from build123d import *

# Parameters (mm, degrees)
BOSS_EXTRUDE1_DEPTH = 40
SKETCH2_W           = 104
SKETCH2_H           = 30
BOSS_EXTRUDE2_DEPTH = 80
BOSS_EXTRUDE3_START = -120
BOSS_EXTRUDE3_DEPTH = 40


with BuildPart() as part:
    # Sketch1 → Boss-Extrude1 (new body)
    with BuildSketch(Plane.XY):
        with BuildLine():
            Line((-52, 0), (-52, -120))
            Line((-52, -120), (52, -120))
            Line((52, -120), (52, 0))
            Line((52, 0), (48, 0))
            ThreePointArc((48, 0), (0, -48), (-48, 0))
            Line((-48, 0), (-52, 0))
        make_face()
    extrude(amount=BOSS_EXTRUDE1_DEPTH)

    # Sketch2 → Boss-Extrude2 (add)
    with BuildSketch(Plane(origin=(0, 0, 0), x_dir=(-1, 0, 0), z_dir=(0, 0, -1))):
        with Locations((0, -105)):
            Rectangle(SKETCH2_W, SKETCH2_H)
    extrude(amount=BOSS_EXTRUDE2_DEPTH)

    # Sketch1<2> → Boss-Extrude3 (add)
    with BuildSketch(Plane.XY.offset(BOSS_EXTRUDE3_START)):
        with BuildLine():
            Line((-52, 0), (-52, -120))
            Line((-52, -120), (52, -120))
            Line((52, -120), (52, 0))
            Line((52, 0), (48, 0))
            ThreePointArc((48, 0), (0, -48), (-48, 0))
            Line((-48, 0), (-52, 0))
        make_face()
    extrude(amount=BOSS_EXTRUDE3_DEPTH)


solid = part.part
Read the model definition and answer for the solid it produces. Units are mm, in the model's axes. A direction names the side the tool comes from. Give positions to 0.01 mm unless a question says otherwise; leave off trailing zeros. Loops run counter-clockwise (first coordinate to the right, second up) from the corner with the lowest first, then second, coordinate; pieces in that order, holes last. Notation, with made-up numbers: M 81.25,46.5 L 108.25,46.5 A29 cw 108.25,84.5 Z; hole C 28,73.25 d5. An arc over 180 degrees is marked long. Write each question's results on one line, items separated by ' | '.
1. The mould has two halves that part along X. Classify faces 1 (the face through (1.06, -47.99, -100.28)), 2 (the face through (50, 0, -100)), 3 (the face through (-52, -99, -41)), 4 (the face through (52, -101, -41)): pulls with the +X half, pulls with the -X half, needs draft (parallel to the pull), parting line crosses it, or undercut.
Values:
face 1: undercut | face 2: needs draft | face 3: pulls with the -X half | face 4: pulls with the +X half
2. Section C-C on x = 0 is taken. Give the vertices of the cut face in (y, z).
Values:
outline: M -120,-120 L -48,-120 L -48,-80 L -90,-80 L -90,0 L -48,0 L -48,40 L -120,40 Z
3. Given pin 1 (12 mm diameter, centred on x = -15.5, z = -17, fed in from +Y), flat-ended and moving along its own axis, determine where the tip first touches the part or whether it passes through.
Values:
pin 1: stops at y = -90
4. Straight lines are drawn through the part: line 1 (Z direction, x = 21, y = -78.5); line 2 (Y direction, x = -2, z = 15); line 3 (Y direction, x = -36, z = -29.5). For each, find the intervals that lie inside material, in ascending order. Write a range as [from, to].
Values:
line 1: z = [-120, -80], [0, 40] | line 2: y = [-120, -47.96] | line 3: y = [-120, -90]
5. Section B-B on y = -45.5 is taken. Give the vertices of the cut face in (x, z).
Values:
outline: M -52,-120 L -15.29,-120 L -15.29,-80 L -52,-80 Z; M -52,0 L -15.29,0 L -15.29,40 L -52,40 Z; M 15.29,-120 L 52,-120 L 52,-80 L 15.29,-80 Z; M 15.29,0 L 52,0 L 52,40 L 15.29,40 Z
6. Section A-A on y = -81 is taken. Give the vertices of the cut face in (x, z).
Values:
outline: M -52,-120 L 52,-120 L 52,-80 L -52,-80 Z; M -52,0 L 52,0 L 52,40 L -52,40 Z
7. A tool of negligible diameter and unlimited length cuts with its end or side. For faces 5 (the face through (-1, -64, -80)), 6 (the face through (-50, 0, 20)), from which of +Z, -Z, +X, -X, +Y, -Y can it reach the whole face along a straight path? Write none if from no direction.
Values:
face 5: +X, -X, +Y | face 6: +Z, -Z, +X, -X, +Y
8. Section D-D on z = 15.5 is taken. Give the vertices of the cut face in (x, y), plus the area to 3 significant figures.
Values:
outline: M -52,-120 L 52,-120 L 52,0 L 48,0 A48 cw -48,0 L -52,0 Z | area: 8,860 mm^2
